from build123d import *

# Parameters (mm, degrees)
SKETCH1_R           = 75
BOSS_EXTRUDE1_DEPTH = 114
SKETCH2_R           = 65
CUT_EXTRUDE1_DEPTH  = 120
SKETCH3_W           = 50
SKETCH3_H           = 15
CUT_EXTRUDE2_DEPTH  = 15


with BuildPart() as part:
    # Sketch1 → Boss-Extrude1 (new body)
    with BuildSketch(Plane(origin=(0, 0, 0), x_dir=(1, 0, 0), z_dir=(0, 1, 0))):
        with Locations(Location((0, 0, 0), (0, 0, 90))):
            Circle(SKETCH1_R)
    extrude(amount=BOSS_EXTRUDE1_DEPTH)

    # Sketch2 → Cut-Extrude1 (cut)
    with BuildSketch(Plane(origin=(0, 114, 0), x_dir=(1, 0, 0), z_dir=(0, 1, 0))):
        with Locations(Location((0, 0, 0), (0, 0, 270))):
            Circle(SKETCH2_R)
    extrude(amount=-CUT_EXTRUDE1_DEPTH, mode=Mode.SUBTRACT)

    # Sketch3 → Cut-Extrude2 (cut)
    with BuildSketch(Plane(origin=(37.49973472, 0, 64.951445805), x_dir=(0.8660254037844382, 0, -0.5000000000000011), z_dir=(0.5000000000000011, 6.982962677686268e-15, 0.8660254037844382))):
        with Locations((0, 52.5)):
            Rectangle(SKETCH3_W, SKETCH3_H)
    extrude(amount=-CUT_EXTRUDE2_DEPTH, mode=Mode.SUBTRACT)


solid = part.part
Geometry: final body of the model. Coordinates: model frame, mm. Give positions to 0.01 mm unless a question says otherwise; leave off trailing zeros. Write each loop counter-clockwise with the first axis right and the second up, starting at its lowest first coordinate (ties: lowest second). Pieces come first, ordered by that corner, then holes. Notation, with made-up numbers: M 44.5,24.5 L 52.5,24.5 A14 cw 52.5,49.5 Z; hole C 53.5,84.5 d3. An arc over 180 degrees is marked long. Answer in a Markdown table with one row per item. Add a question column.
(1) Section C-C on x = 24. Return loops of the section in (y, z).
(2) First-contact query: pin 1 (6 mm diameter, centred on x = -14.5, y = 34.5, fed in from -Z); pin 2 (4 mm diameter, centred on x = -7.5, y = 80, fed in from +Z); pin 3 (1.5 mm diameter, centred on y = 63.5, z = 20, fed in from -X). Flat tips, straight axial feed; report the tip coordinate or a pass-through.
(3) Section B-B on z = 0. Return loops of the section in (x, y).
(4) Section D-D on y = 14.5. Return loops of the section in (x, z).
(5) Section A-A on x = 0. Return loops of the section in (y, z), and give its area (3 significant figures).
(6) Ray query, line 1 (X direction, y = 57, z = 0); line 2 (X direction, y = 103, z = 4.5); line 3 (Z direction, x = -31, y = 43). Return the intervals inside material, ascending.
(7) Mould query, pull axis Y, two halves, no side actions, for faces 1 (the flat face through (54.366, 52.395, 44.164)), 2 (the flat face through (-61, 114, 23)), 3 (the flat face through (-61, 0, 23)), 4 (the flat face through (34, 60, 60)). Classes: +Y half, -Y half, draft (parallel to the pull), parting line (faces both ways), or undercut.
Result set:
| question | item | result |
|---|---|---|
| 1 | outline | M 0,-71.06 L 114,-71.06 L 114,-60.41 L 0,-60.41 Z; M 0,60.41 L 45,60.41 L 45,71.06 L 0,71.06 Z; M 60,60.41 L 114,60.41 L 114,71.06 L 60,71.06 Z |
| 2 | pin 1 | stops at z = -74.11 |
| 2 | pin 2 | stops at z = 74.8 |
| 2 | pin 3 | stops at x = -72.49 |
| 3 | outline | M -75,0 L -65,0 L -65,114 L -75,114 Z; M 65,0 L 75,0 L 75,114 L 65,114 Z |
| 4 | outline | C 0,0 d150; hole C 0,0 d130 |
| 5 | outline | M 0,-75 L 114,-75 L 114,-65 L 0,-65 Z; M 0,65 L 114,65 L 114,75 L 0,75 Z |
| 5 | area | 2,280 mm^2 |
| 6 | line 1 | x = -75 to -65, 65 to 75 |
| 6 | line 2 | x = -74.86 to -64.84, 64.84 to 74.86 |
| 6 | line 3 | z = -68.29 to -57.13, 57.13 to 68.29 |
| 7 | face 1 | undercut |
| 7 | face 2 | +Y half |
| 7 | face 3 | -Y half |
| 7 | face 4 | undercut |
